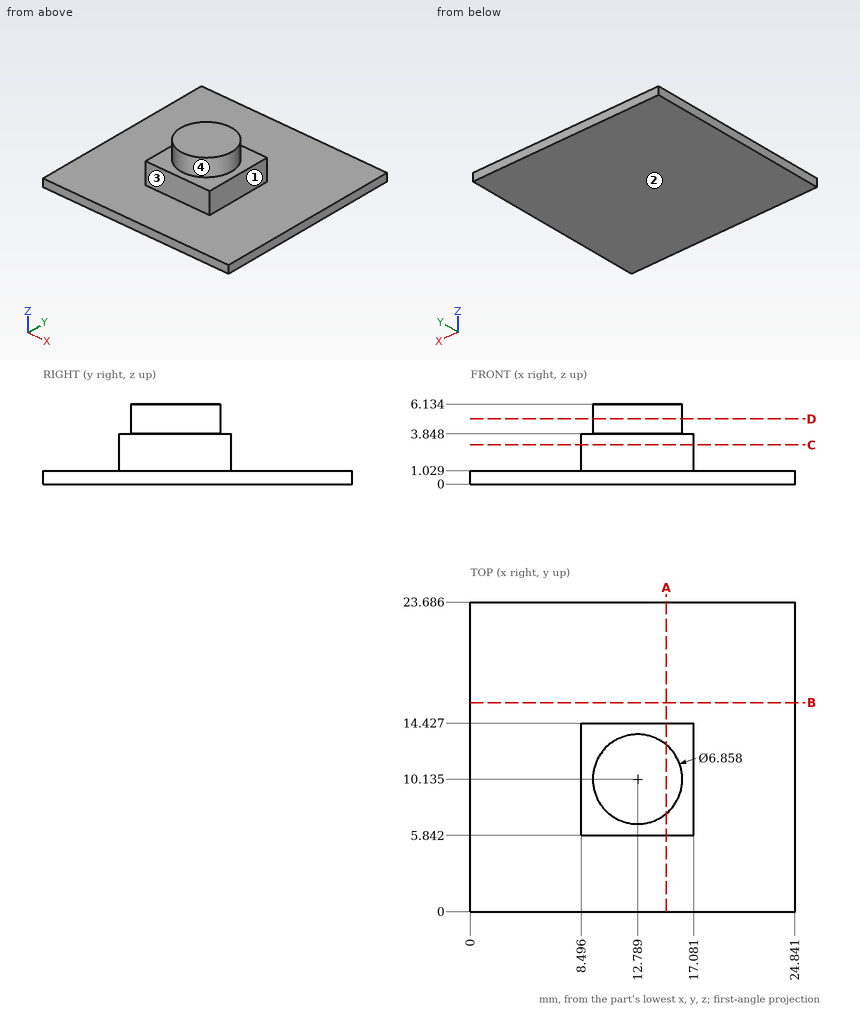
Can you work these out from the drawing? Everything is in mm from the part's minimum corner. A direction names the side the tool comes from. Give positions to 0.01 mm unless a question says otherwise; leave off trailing zeros. Order: outer loops, then holes, each group sorted by start corner. A loop starts at its lowest first (then second) coordinate and runs counter-clockwise, first axis right, second up. Notation, with made-up numbers: M 49.25,55.5 L 89.25,55.5 A19 cw 89.25,72.5 Z; hole C -4,13.5 d6. An arc over 180 degrees is marked long. Write item = value, one per line. Start each with the question number.
Q1. Suppose I cut it at C-C (z = 3). Write out the boundary of the cut face in (x, y).
Q2. I need wall thicknesses on probe 1 along Z at (x, y) = (21, 13.75); probe 2 along X at (y, z) = (11.25, 2.25); probe 3 along Y at (x, z) = (15.75, 2.5). Which ranges of each line are inside material? Lowest first, please. Write a range as [from, to].
Q3. Will these pins go through, and if not, where does the flat tip stop? pin 1 Ø1 at (y, z) = (16, 2) entering from -X; pin 2 Ø2.5 at (x, z) = (14, 3) entering from +Y; pin 3 Ø5 at (x, y) = (20.5, 20) entering from +Z; pin 4 Ø10 at (x, y) = (5, 6.5) entering from +Z.
Q4. Suppose I cut it at B-B (y = 16). Write out the boundary of the cut face in (x, z).
Q5. Suppose I cut it at D-D (z = 5). Write out the boundary of the cut face in (x, y) (1 decimal).
Q6. Suppose I cut it at A-A (x = 15). Write out the boundary of the cut face in (y, z) (1 decimal).
Q7. For the marked faces 1, 2, 3 and 4, which set-ups out of +Z, -Z, +X, -X, +Y, -Y let a thin tool reach every point of the face, with its end or its side?
Check result:
q1.outline = M 8.5,5.84 L 17.08,5.84 L 17.08,14.43 L 8.5,14.43 Z
q2.probe_1 = [0, 1.03]
q2.probe_2 = [8.5, 17.08]
q2.probe_3 = [5.84, 14.43]
q3.pin_1 = through
q3.pin_2 = 14.43
q3.pin_3 = 1.03
q3.pin_4 = 3.85
q4.outline = M 0,0 L 24.84,0 L 24.84,1.03 L 0,1.03 Z
q5.outline = C 12.8,10.1 d6.9
q6.outline = M 0,0 L 23.7,0 L 23.7,1 L 14.4,1 L 14.4,3.8 L 12.8,3.8 L 12.8,6.1 L 7.5,6.1 L 7.5,3.8 L 5.8,3.8 L 5.8,1 L 0,1 Z
q7.face_1 = +Z, +X, +Y, -Y
q7.face_2 = -Z, +X, -X, +Y, -Y
q7.face_3 = +Z, +X, -X, -Y
q7.face_4 = +Z
